Could you check a few things on this model? Use its own coordinates, in mm. A direction names the side the tool comes from. Coordinates: 2 decimals unless noted, no trailing zeros. Write each loop counter-clockwise with the first axis right and the second up, starting at its lowest first coordinate (ties: lowest second). Pieces come first, ordered by that corner, then holes. Notation, with made-up numbers: M 65,46.5 L 72,46.5 A23 cw 72,65.5 Z; hole C 19.25,88.5 d3. An arc over 180 degrees is marked long. Write item = value, one per line.
```python
from build123d import *

# Parameters (mm, degrees)
SKETCH1_W           = 200
SKETCH1_H           = 205
BOSS_EXTRUDE1_DEPTH = 10
SKETCH2_W           = 10
SKETCH2_H           = 15
BOSS_EXTRUDE2_DEPTH = 160
SKETCH4_W           = 50
SKETCH4_H           = 10
BOSS_EXTRUDE3_DEPTH = 15
SKETCH5_W           = 45
SKETCH5_H           = 10
BOSS_EXTRUDE4_DEPTH = 15
SKETCH6_R           = 2
CUT_EXTRUDE1_DEPTH  = 15
SKETCH10_R          = 1
CUT_EXTRUDE2_DEPTH  = 5
CUT_EXTRUDE3_START  = 5
SKETCH7_R           = 1
CUT_EXTRUDE3_DEPTH  = 5


with BuildPart() as part:
    # Sketch1 → Boss-Extrude1 (new body)
    with BuildSketch(Plane(origin=(0, 0, 0), x_dir=(1, 0, 0), z_dir=(0, 1, 0))):
        Rectangle(SKETCH1_W, SKETCH1_H)
    extrude(amount=BOSS_EXTRUDE1_DEPTH)

    # Sketch2 → Boss-Extrude2 (add)
    with BuildSketch(Plane(origin=(0, 0, 0), x_dir=(1, 0, 0), z_dir=(0, 1, 0))):
        with Locations((-20, -95)):
            Rectangle(SKETCH2_W, SKETCH2_H)
        with Locations((20, -95)):
            Rectangle(SKETCH2_W, SKETCH2_H)
    extrude(amount=BOSS_EXTRUDE2_DEPTH)

    # Sketch4 → Boss-Extrude3 (add)
    with BuildSketch(Plane.XY.offset(102.5)):
        with Locations((0, 145)):
            Rectangle(SKETCH4_W, SKETCH4_H)
    extrude(amount=BOSS_EXTRUDE3_DEPTH)

    # Sketch5 → Boss-Extrude4 (add)
    with BuildSketch(Plane.XY.offset(117.5)):
        with Locations((-0.452584592, 145)):
            Rectangle(SKETCH5_W, SKETCH5_H)
    extrude(amount=BOSS_EXTRUDE4_DEPTH)

    # Sketch6 → Cut-Extrude1 (cut)
    with BuildSketch(Plane(origin=(0, 150, 0), x_dir=(1, 0, 0), z_dir=(0, 1, 0))):
        with Locations(Location((-14.952584592, -125, 0), (0, 0, 270))):
            Circle(SKETCH6_R)
        with Locations(Location((14.047415408, -125, 0), (0, 0, 270))):
            Circle(SKETCH6_R)
    extrude(amount=-CUT_EXTRUDE1_DEPTH, mode=Mode.SUBTRACT)

    # Sketch10 → Cut-Extrude2 (cut)
    with BuildSketch(Plane(origin=(-15, 0, 0), x_dir=(0, 0, -1), z_dir=(1, 0, 0))):
        with Locations((-95, 150)):
            Circle(SKETCH10_R)
    extrude(amount=-CUT_EXTRUDE2_DEPTH, mode=Mode.SUBTRACT)

    # Sketch7 → Cut-Extrude3 (cut)
    with BuildSketch(Plane(origin=(15, 0, 0), x_dir=(0, 0, -1), z_dir=(1, 0, 0)).offset(CUT_EXTRUDE3_START)):
        with Locations((-95, 150)):
            Circle(SKETCH7_R)
    extrude(amount=-CUT_EXTRUDE3_DEPTH, mode=Mode.SUBTRACT)


solid = part.part
```
Item 1: If we mould it in two halves opening along X, with no side actions, what happens to faces 4 (the face through (-100, 5, 1)), 5 (the face through (-15, 84, 95)), 6 (the face through (20, 84, 87.5))? For each: pulls with the +X half, pulls with the -X half, needs draft (parallel to the pull), parting line crosses it, or undercut.
Numbers:
face_4 = pulls with the -X half
face_5 = undercut
face_6 = needs draft
Item 2: Imagine slicing it at B-B (x = 2.5). Write out the boundary of the cut face in (y, z).
Numbers:
outline = M 0,-102.5 L 10,-102.5 L 10,102.5 L 0,102.5 Z; M 140,102.5 L 150,102.5 L 150,132.5 L 140,132.5 Z
Item 3: Imagine slicing it at C-C (x = 49). Write out the boundary of the cut face in (y, z).
Numbers:
outline = M 0,-102.5 L 10,-102.5 L 10,102.5 L 0,102.5 Z
Item 4: If I drill on line 1 along X through (y, z) = (145, 125); line 2 along X through (y, z) = (56, 94.5); line 3 along Z through (x, y) = (22, 72), over which ranges is the centre line in solid material (lowest first)?
Numbers:
line_1 = -22.95 to -16.95, -12.95 to 12.05, 16.05 to 22.05
line_2 = -25 to -15, 15 to 25
line_3 = 87.5 to 102.5
Item 5: Imagine slicing it at A-A (y = 20). Write out the boundary of the cut face in (x, z), and give its area (3 significant figures).
Numbers:
outline = M -25,87.5 L -15,87.5 L -15,102.5 L -25,102.5 Z; M 15,87.5 L 25,87.5 L 25,102.5 L 15,102.5 Z
area = 300 mm²
Item 6: Imagine slicing it at D-D (z = -9). Write out the boundary of the cut face in (x, y), and give its area (3 significant figures).
Numbers:
outline = M -100,0 L 100,0 L 100,10 L -100,10 Z
area = 2,000 mm²
Item 7: For faces 1 (the face through (-20, 155, 102.5)), 2 (the face through (25, 84, 96)), 3 (the face through (22.047, 145, 125)), which set-ups out of +Z, -Z, +X, -X, +Y, -Y let a thin tool reach every point of the face, with its end or its side?
Numbers:
face_1 = +Z, +X, -X, +Y
face_2 = +Z, -Z, +X, +Y
face_3 = +Z, +X, +Y, -Y
Item 8: I'm going to push flat-ended pins straight in: P1, Ø16.5, axis at y = 72, z = 97.5, coming from the +X side; P2, Ø5, axis at y = 41, z = 100, coming from the -X side; P3, Ø3, axis at y = 146.5, z = 125.5, coming from the +X side. Where does each tip first touch, or does it pass through?
Numbers:
P1 = 25
P2 = -25
P3 = 22.05
